from build123d import *

# Parameters (mm, degrees)
F2_SIZE       = 0.79375
F3_W          = 1.5
F3_H          = 6.0875
F4_DEPTH      = 4.001
F4_DEPTH_BACK = 4.001
F5_T4_DEPTH   = 7.1310276602
F5_S5_R       = 1.75
F5_T6_DEPTH   = 5
F5_T10_DEPTH  = 7.1310276602
F5_S11_R      = 1.75
F5_T12_DEPTH  = 5
F6_R          = 0.5


# Not quite as in the source:
# - a fillet or chamfer that OpenCascade refuses, or shapes differently, is made with other operations: its cross-section is extruded or revolved along the edge and cut away or added


with BuildPart() as f1:
    # F0 (on Front) → F1 (revolve)
    with BuildSketch(Plane.XZ):
        Polygon((4, 0), (1.75, 0), (1.75, 5), (2.5, 5), (2.5, 6.5875), (0, 6.5875), (0, 5), (0, 0), (0, -1), (4, -1), align=None)
    revolve(axis=Axis((0, 0, 2.5), (0, 0, 1)))

    # F2
    f2_edges = [f1.edges().sort_by_distance(p)[0] for p in [
        (-2.5, 0, 6.5875),
    ]]
    chamfer(f2_edges, length=F2_SIZE)

    # F3 (on Front) → F4 (cut, two sides)
    with BuildSketch(Plane.XZ) as f4_sk:
        with Locations((0, 3.54375)):
            Rectangle(F3_W, F3_H)
    extrude(amount=F4_DEPTH, mode=Mode.SUBTRACT)
    extrude(f4_sk.sketch, amount=-F4_DEPTH_BACK, mode=Mode.SUBTRACT)

    # F5: fillet of radius 0.79375 on 2 edges, made by hand


with BuildPart() as f5_tool2:
    # F5_s3 → F5_t4 (new body)
    with BuildSketch(Plane.XZ.offset(-3.5655138301)):
        with BuildLine():
            ThreePointArc((-0.04375, 0.5), (0.5175160076, 0.7324839924), (0.75, 1.29375))
            Line((0.75, 1.29375), (0.75, 0.5))
            Line((0.75, 0.5), (-0.04375, 0.5))
        make_face()
    extrude(amount=F5_T4_DEPTH)

    # F5_s5 → F5_t6 (intersect, symmetric)
    with BuildSketch(Plane.XY.offset(0.9)):
        Circle(F5_S5_R)
    extrude(amount=F5_T6_DEPTH, both=True, mode=Mode.INTERSECT)


with BuildPart() as f1_1:
    add(f1.part)

    # F5_t1: union F5_tool2
    add(f5_tool2.part)


with BuildPart() as f5_tool8:
    # F5_s9 → F5_t10 (new body)
    with BuildSketch(Plane.XZ.offset(-3.5655138301)):
        with BuildLine():
            ThreePointArc((-0.75, 1.29375), (-0.5175160076, 0.7324839924), (0.04375, 0.5))
            Line((0.04375, 0.5), (-0.75, 0.5))
            Line((-0.75, 0.5), (-0.75, 1.29375))
        make_face()
    extrude(amount=F5_T10_DEPTH)

    # F5_s11 → F5_t12 (intersect, symmetric)
    with BuildSketch(Plane.XY.offset(0.9)):
        Circle(F5_S11_R)
    extrude(amount=F5_T12_DEPTH, both=True, mode=Mode.INTERSECT)


with BuildPart() as f1_2:
    add(f1_1.part)

    # F5_t7: union F5_tool8
    add(f5_tool8.part)

    # F6
    f6_edges = [f1_2.edges().sort_by_distance(p)[0] for p in [
        (-4, 0, -1),
    ]]
    fillet(f6_edges, radius=F6_R)


solid = f1_2.part
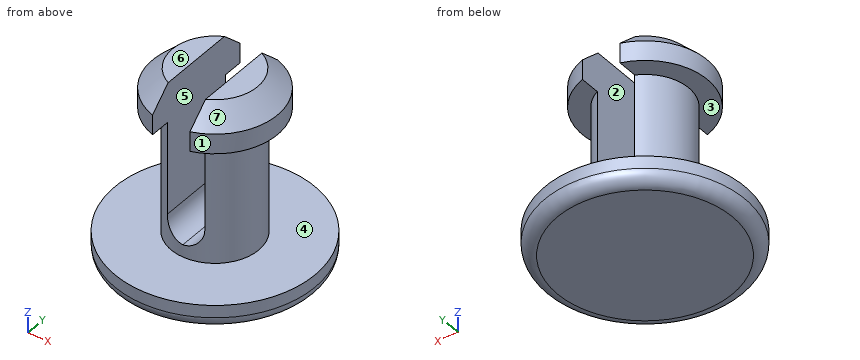
Part model, mm, in its own coordinate system. Face numbers are marked on the shaded views. A direction names the side the tool comes from. Coordinates: 2 decimals unless noted, no trailing zeros. Order: outer loops, then holes, each group sorted by start corner. A loop starts at its lowest first (then second) coordinate and runs counter-clockwise, first axis right, second up. Notation, with made-up numbers: (72.5, 8) - (108.5, 8) arc R28 ccw to (108.5, 27) - close; hole circle Ø5 at (51, 42.25). An arc over 180 degrees is marked (long way). Use CSV: the item, a comma, the result in double quotes.
Item 1: Saw through at B-B on z = 3. Give the cut face in (x, y), and give its area (3 significant figures).
Solved:
outline,"(-0.75, -1.58) - (-0.75, 1.58) arc R1.75 ccw to start; (0.75, -1.58) arc R1.75 ccw to (0.75, 1.58) - close"
area,"4.54 mm²"
Item 2: Saw through at C-C on y = 2. Give the number of separate pieces and of enclosed holes in the cut face, and give its area (3 significant figures).
Solved:
separate pieces,"3"
enclosed holes,"0"
area,"8.29 mm²"
Item 3: 3-axis set-ups, long thin cutter, end or side, ignore diameter. For the marked faces 1, 2, 3 and 4: which of +Z, -Z, +X, -X, +Y, -Y reach the whole face in a straight line?
Solved:
face 1,"+Z, +X"
face 2,"+Z, +Y, -Y"
face 3,"-X"
face 4,"none"
Item 4: Mould opens along X. For the marked faces 5, 6 and 7 say: +X half, -X half, draft (parallel to the pull), parting line (faces both ways), or undercut.
Solved:
face 5,"undercut"
face 6,"draft"
face 7,"+X half"
Item 5: Saw through at A-A on y = 0. Give the cut face in (x, z).
Solved:
outline,"(-4, -0.5) arc R0.5 ccw to (-3.5, -1) - (3.5, -1) arc R0.5 ccw to (4, -0.5) - (4, 0) - (1.75, 0) - (1.75, 5) - (2.5, 5) - (2.5, 5.79) - (1.71, 6.59) - (0.75, 6.59) - (0.75, 1.29) arc R0.79 cw to (0, 0.5) arc R0.79 cw to (-0.75, 1.29) - (-0.75, 6.59) - (-1.71, 6.59) - (-2.5, 5.79) - (-2.5, 5) - (-1.75, 5) - (-1.75, 0) - (-4, 0) - close"
Item 6: Probe probe 1 along X at (y, z) = (-0.75, 5.25); probe 2 along X at (y, z) = (0, 5.25); probe 3 along Z at (x, y) = (-1.75, -2). List the from-to ranges inside material, lowest first.
Solved:
probe 1,"x = -2.38 to -0.75, 0.75 to 2.38"
probe 2,"x = -2.5 to -0.75, 0.75 to 2.5"
probe 3,"z = -1 to 0"
Item 7: Drop flat-ended pins along their axis: P1, Ø4, axis at y = 1, z = 4, coming from the +X side; P2, Ø2.5, axis at y = 0, z = 3, coming from the -X side; P3, Ø2, axis at x = -1, z = 4.5, coming from the -Y side. Give the stop position or say it passes through.
Solved:
P1,"stops at x = 2.5"
P2,"stops at x = -1.75"
P3,"stops at y = -2.38"
